```python
from build123d import *

# Parameters (mm, degrees)
SKETCH1_R                  = 60
BOSS_EXTRUDE1_DEPTH        = 100
M8_CLEARANCE_HOLE1_D       = 10
F_10_0MM_DOWEL_HOLE1_D     = 10
F_10_0MM_DOWEL_HOLE1_DEPTH = 8
F_10_0MM_DOWEL_HOLE1_TIP   = 3.004303095


with BuildPart() as part:
    # Sketch1 → Boss-Extrude1 (new body)
    with BuildSketch(Plane(origin=(0, 0, 0), x_dir=(1, 0, 0), z_dir=(0, 1, 0))):
        with BuildLine():
            Line((-100, -75), (100, -75))
            Line((100, -75), (100, -58.4))
            Line((100, -58.4), (78.5, -58.4))
            Line((78.5, -58.4), (78.5, 0))
            Line((78.5, 0), (78.5, 43.8))
            Line((78.5, 43.8), (60.881524291, 43.8))
            ThreePointArc((60.881524291, 43.8), (0, 75), (-60.881524291, 43.8))
            Line((-60.881524291, 43.8), (-78.5, 43.8))
            Line((-78.5, 43.8), (-78.5, 0))
            Line((-78.5, 0), (-78.5, -58.4))
            Line((-78.5, -58.4), (-100, -58.4))
            Line((-100, -58.4), (-100, -75))
        make_face()
        with Locations(Location((0, 0, 0), (0, 0, 270))):
            Circle(SKETCH1_R, mode=Mode.SUBTRACT)
    extrude(amount=BOSS_EXTRUDE1_DEPTH)

    # M8 Clearance Hole1 (through all)
    with Locations(Plane.XY.offset(75)):
        with Locations((-90, 80), (-90, 20), (90, 20), (90, 80)):
            Hole(M8_CLEARANCE_HOLE1_D / 2)

    # Ø10.0mm Dowel Hole1
    with Locations(Plane.XY.offset(75)):
        with Locations((0, 50)):
            Hole(F_10_0MM_DOWEL_HOLE1_D / 2, depth=F_10_0MM_DOWEL_HOLE1_DEPTH)
            with Locations((0, 0, -(F_10_0MM_DOWEL_HOLE1_DEPTH + F_10_0MM_DOWEL_HOLE1_TIP / 2))):  # 118° drill point
                Cone(0, F_10_0MM_DOWEL_HOLE1_D / 2, F_10_0MM_DOWEL_HOLE1_TIP, mode=Mode.SUBTRACT)


solid = part.part
```
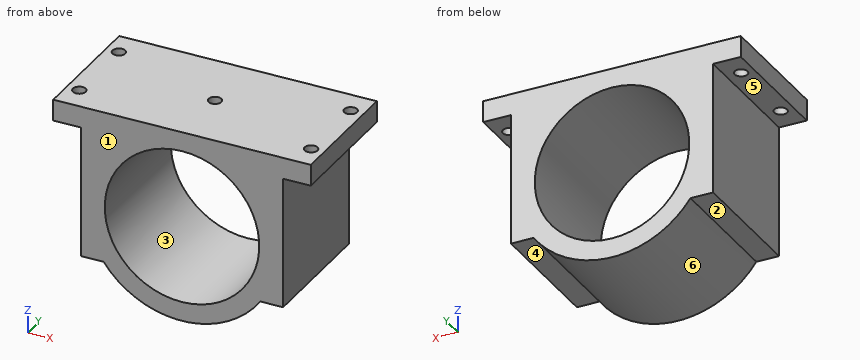
The listing builds one solid part. Answer for the finished solid, in the listing's coordinates (mm). Face numbers are marked on the shaded views. A direction names the side the tool comes from. Round coordinates to 2 decimals unless told otherwise and drop trailing zeros. Loops run counter-clockwise (first coordinate to the right, second up) from the corner with the lowest first, then second, coordinate; pieces in that order, holes last.
1) A cutting plane is placed at D-D on x = 41. Determine the outline of the cut face in (y, z).
Outcome:
outline: (0, -62.8) - (100, -62.8) - (100, -43.81) - (0, -43.81) - close; (0, 43.81) - (100, 43.81) - (100, 75) - (0, 75) - close
2) Given P1, Ø5.5, axis at x = 74, y = 73.5, coming from the -Z side; P2, Ø8, axis at x = -90, y = 20, coming from the +Z side; P3, Ø12, axis at y = 80.5, z = 2, coming from the +X side; P4, Ø1, axis at y = 47.5, z = -19, coming from the -X side, each flat-ended and moving along its own axis, determine where each tip first touches the part or whether it passes through.
Outcome:
P1: stops at z = -43.8
P2: passes through
P3: stops at x = 78.5
P4: stops at x = -78.5
3) For a pull along Z with two mould halves and no side action, classify the marked faces 1, 2 and 3 as released by +Z, released by -Z, zero draft, split by the parting line, or undercut.
Outcome:
face 1: zero draft
face 2: released by -Z
face 3: undercut
4) A cutting plane is placed at C-C on z = 7.5. Determine the outline of the cut face in (x, y).
Outcome:
outline: (-78.5, 0) - (-59.53, 0) - (-59.53, 100) - (-78.5, 100) - close; (59.53, 0) - (78.5, 0) - (78.5, 100) - (59.53, 100) - close
5) A cutting plane is placed at A-A on y = 20. Determine the outline of the cut face in (x, z).
Outcome:
outline: (-100, 58.4) - (-95, 58.4) - (-95, 75) - (-100, 75) - close; (-85, 58.4) - (-78.5, 58.4) - (-78.5, -43.8) - (-60.88, -43.8) arc R75 ccw to (60.88, -43.8) - (78.5, -43.8) - (78.5, 58.4) - (85, 58.4) - (85, 75) - (-85, 75) - close; (95, 58.4) - (100, 58.4) - (100, 75) - (95, 75) - close; hole circle Ø120 at (0, 0)
6) For the marked faces 4, 5 and 6, determine the directions among +Z, -Z, +X, -X, +Y, -Y from which every point of the face is accessible in a straight line to the end or side of a thin tool.
Outcome:
face 4: -Z, +X, +Y, -Y
face 5: -Z, -X, +Y, -Y
face 6: -Z, +Y, -Y
7) Consider line 1 (Y direction, x = 90, z = 65.5); line 2 (X direction, y = 50, z = 73); line 3 (X direction, y = 78, z = 0). Determine where each line is inside the solid, lowest interval first.
Outcome:
line 1: y = 0 to 15, 25 to 75, 85 to 100
line 2: x = -100 to -5, 5 to 100
line 3: x = -78.5 to -60, 60 to 78.5
8) A cutting plane is placed at B-B on x = 90. Determine the outline of the cut face in (y, z), plus the area to 3 significant figures.
Outcome:
outline: (0, 58.4) - (15, 58.4) - (15, 75) - (0, 75) - close; (25, 58.4) - (75, 58.4) - (75, 75) - (25, 75) - close; (85, 58.4) - (100, 58.4) - (100, 75) - (85, 75) - close
area: 1,330 mm2
